Geometry: final body of the model. Coordinates: model frame, mm. A direction names the side the tool comes from. Round coordinates to 2 decimals unless told otherwise and drop trailing zeros. Loops run counter-clockwise (first coordinate to the right, second up) from the corner with the lowest first, then second, coordinate; pieces in that order, holes last. Notation, with made-up numbers: (44.5, 13) - (94.5, 13) arc R31 ccw to (94.5, 45) - close; hole circle Ø9 at (86.25, -38). An arc over 180 degrees is marked (long way). Use CSV: the item, a comma, the result in double quotes.
Autodesk Inventor part; units mm, degrees
ref_plane "YZ Plane" through (0, 0, 0) normal (1, 0, 0) x (0, 1, 0)
ref_plane "XZ Plane" through (0, 0, 0) normal (0, 1, 0) x (-1, 0, 0)
ref_plane "XY Plane" through (0, 0, 0) normal (0, 0, 1) x (1, 0, 0)
sketch "Sketch1" plane through (0, 0, 0) normal (0, 0, 1) x (1, 0, 0)
  arc A0 (-21.082, 52.832) -> (21.082, 52.832) centre (0, 52.832) ccw
  line L0 (-21.082, 52.832) -> (-21.082, 0)
  line L1 (21.082, 52.832) -> (21.082, 0)
  line L2 (-21.082, 0) -> (21.082, 0)
  line L3 (-21.082, 0) -> (-27.432, 0)
  line L4 (-27.432, 0) -> (-27.432, 82.55)
  line L5 (-27.432, 82.55) -> (-24.257, 82.55)
  line L6 (-21.082, 79.375) -> (-21.082, 0)
  line L7 (21.082, 0) -> (27.432, 0)
  line L8 (27.432, 0) -> (27.432, 82.55)
  line L9 (27.432, 82.55) -> (24.257, 82.55)
  line L10 (21.082, 79.375) -> (21.082, 0)
  line L11 (0, 0) -> (-27.432, 0) construction
  arc A1 (24.257, 82.55) -> (21.082, 79.375) centre (24.257, 79.375) ccw
  arc A2 (-21.082, 79.375) -> (-24.257, 82.55) centre (-24.257, 79.375) ccw
  point P0 (-21.082, 82.55)
  point P1 (21.082, 82.55)
  dimension "diameterOfPipe" = 42.164
  dimension "d6" = 6.35
  dimension "d8" = 6.35
  dimension "d27" = 82.55
  dimension "d28" = 52.832
  dimension "d29" = 31.75
  dimension "d30" = 3.175
revolve "Revolution1" add sketch "Sketch1" angle 360 about axis through (-21.082, 0, 0) along (1, 0, 0)
sketch "Sketch3" plane through (27.432, 0, 0) normal (1, 0, 0) x (0, 0, -1)
  line L0 (7.9189, 0) -> (3.9595, -6.858)
  line L1 (3.9595, -6.858) -> (-3.9595, -6.858)
  line L2 (-3.9595, -6.858) -> (-7.9189, 0)
  line L3 (-7.9189, 0) -> (-3.9595, 6.858)
  line L4 (-3.9595, 6.858) -> (3.9595, 6.858)
  line L5 (3.9595, 6.858) -> (7.9189, 0)
  point P0 (0, 0)
  point P1 (0, 0)
  dimension "hexWidth" = 13.716
extrude "Extrusion2" cut sketch "Sketch3" against normal through all
sketch "Sketch4" plane through (27.432, 0, 0) normal (1, 0, 0) x (0, 0, -1)
  point P0 (0, 0)
  point P1 (0, 25.4)
  point P2 (-21.997, 12.7)
  point P3 (-21.997, -12.7)
  point P4 (0, -25.4)
  point P5 (21.997, -12.7)
  point P6 (21.997, 12.7)
  dimension "d14" = 25.4
  dimension "d17" = 360
hole "Hole1" at (27.432, 25.4, 0) at (27.432, 12.7, 21.997) at (27.432, -12.7, 21.997) at (27.432, -25.4, 0) at (27.432, -12.7, -21.997) at (27.432, 12.7, -21.997) direction (-1, 0, 0) diameter 5.1054 end through all
equation "\"widthOfOutside\" = 6.35"
properties part number "WheelForHangingAndMoving" material "PBT Plastic"
Item 1: Reachability of faces 5 (the flat face through (21.082, 52, -17)), 6 (the flat face through (0.4, -3.5, 5.9)) from +Z, -Z, +X, -X, +Y, -Y: full face, straight path, thin tool, end or side. Return the list, or none.
Final values:
face 5,"none"
face 6,"+X, -X"
Item 2: Pin query (flat end, axial travel): P1, Ø6.5, axis at y = -25.4, z = 0, coming from the -X side; P2, Ø2.5, axis at x = 11.5, z = 1, coming from the -Y side; P3, Ø1, axis at x = 12.5, z = -0.5, coming from the -Y side; P4, Ø10, axis at x = 4, z = 8, coming from the -Y side. Return the tip coordinate at first contact, or that it passes through.
Final values:
P1,"stops at x = -27.43"
P2,"stops at y = -36.03"
P3,"stops at y = -36.23"
P4,"stops at y = -33.04"
Item 3: Mould query, pull axis X, two halves, no side actions, for faces 1 (the cylindrical face through (25.822, -17.895, 80.587)), 2 (the flat face through (-21.082, 52, -17)), 3 (the flat face through (27.432, -1, -17)), 4 (the flat face through (-27.432, -1, -17)). Classes: released by +X, released by -X, zero draft, split by the parting line, or undercut.
Final values:
face 1,"zero draft"
face 2,"undercut"
face 3,"released by +X"
face 4,"released by -X"
Item 4: Section C-C on y = 12.7. Give the number of separate pieces and of enclosed holes in the cut face, plus the area to 3 significant figures.
Final values:
separate pieces,"3"
enclosed holes,"0"
area,"4,360 mm²"
Item 5: Material intervals for line 1 (X direction, y = 69, z = 22); line 2 (Z direction, x = 25, y = -14); line 3 (Z direction, x = 25.5, y = 11.5), sorted ascending.
Final values:
line 1,"x = -27.43 to -21.08, 21.08 to 27.43"
line 2,"z = -81.35 to -24.19, -19.8 to 19.8, 24.19 to 81.35"
line 3,"z = -81.75 to -24.25, -19.74 to 19.74, 24.25 to 81.75"
Item 6: Section B-B on x = 17.5. Return the cut outline in (y, z).
Final values:
outline,"circle Ø82.15 at (0, 0); hole circle Ø5.11 at (-25.4, 0); hole circle Ø5.11 at (-12.7, -22); hole circle Ø5.11 at (-12.7, 22); hole (-6.86, -3.96) - (0, -7.92) - (6.86, -3.96) - (6.86, 3.96) - (0, 7.92) - (-6.86, 3.96) - close; hole circle Ø5.11 at (12.7, -22); hole circle Ø5.11 at (12.7, 22); hole circle Ø5.11 at (25.4, 0)"
Item 7: Section A-A on x = -17. Return the cut outline in (y, z).
Final values:
outline,"circle Ø80.73 at (0, 0); hole circle Ø5.11 at (-25.4, 0); hole circle Ø5.11 at (-12.7, -22); hole circle Ø5.11 at (-12.7, 22); hole (-6.86, -3.96) - (0, -7.92) - (6.86, -3.96) - (6.86, 3.96) - (0, 7.92) - (-6.86, 3.96) - close; hole circle Ø5.11 at (12.7, -22); hole circle Ø5.11 at (12.7, 22); hole circle Ø5.11 at (25.4, 0)"
